Here's how the part is built. I have some questions about the finished solid (model axes, mm). A direction names the side the tool comes from. Round coordinates to 2 decimals unless told otherwise and drop trailing zeros. Order: outer loops, then holes, each group sorted by start corner. A loop starts at its lowest first (then second) coordinate and runs counter-clockwise, first axis right, second up. Notation, with made-up numbers: (18.25, 35) - (76.25, 35) arc R33 cw to (76.25, 70) - close; hole circle Ø9 at (39, 20). An arc over 180 degrees is marked (long way). One line per item, written item: value.
from build123d import *

# Parameters (mm, degrees)
SKETCH_W        = 40
SKETCH_H        = 40
PAD_DEPTH       = 2
SKETCH001_R     = 10.1
PAD001_DEPTH    = 6
SKETCH002_R     = 8
POCKET_DEPTH    = 6
SKETCH003_W     = 2.007961
SKETCH003_H     = 21.864484
SKETCH003_W_2   = 7.094803
SKETCH003_H_2   = 2.097204
SKETCH003_W_3   = 6.916317
SKETCH003_H_3   = 1.96334
POCKET001_DEPTH = 6
FILLET_R        = 2


with BuildPart() as part:
    # Sketch → Pad (new body)
    with BuildSketch(Plane.XY):
        with Locations((20, -20)):
            Rectangle(SKETCH_W, SKETCH_H)
    extrude(amount=PAD_DEPTH)

    # Sketch001 (on Face6 of Pad) → Pad001 (join)
    with BuildSketch(Plane.XY.offset(2)):
        with Locations((20, -20)):
            Circle(SKETCH001_R)
    extrude(amount=PAD001_DEPTH)

    # Sketch002 (on Face8 of Pad001) → Pocket (cut)
    with BuildSketch(Plane.XY.offset(8)):
        with Locations((20, -20)):
            Circle(SKETCH002_R)
    extrude(amount=-POCKET_DEPTH, mode=Mode.SUBTRACT)

    # Sketch003 (on Face8 of Pocket) → Pocket001 (cut)
    with BuildSketch(Plane.XY.offset(8)):
        with Locations((20.041939, -19.903789)):
            Rectangle(SKETCH003_W, SKETCH003_H)
        with Locations((28.520004, -19.970721)):
            Rectangle(SKETCH003_W_2, SKETCH003_H_2)
        with Locations((12.456301, -20.037653)):
            Rectangle(SKETCH003_W_3, SKETCH003_H_3)
    extrude(amount=-POCKET001_DEPTH, mode=Mode.SUBTRACT)

    # Fillet
    fillet_edges = [part.edges().sort_by_distance(p)[0] for p in [
        (40, -40, 1),
        (40, 0, 1),
        (0, -40, 1),
        (0, 0, 1),
    ]]
    fillet(fillet_edges, radius=FILLET_R)


solid = part.part
Q1. We'd pull the mould along Y, two halves only. Please class faces 1 (the flat face through (14, -26, 8)), 2 (the cylindrical face through (25.697, -14.384, 5.042)), 3 (the cylindrical face through (27.198, -12.915, 4.958)): released by +Y, released by -Y, zero draft, split by the parting line, or undercut.
Results list:
face 1: zero draft
face 2: undercut
face 3: released by +Y
Q2. If I drill on line 1 along Y through (x, z) = (19, 6); line 2 along Z through (x, y) = (3.5, -6.5); line 3 along X through (y, z) = (-14, 4), over which ranges is the centre line in solid material (lowest first)?
Results list:
line 1: -30.05 to -27.94, -12.06 to -9.95
line 2: 0 to 2
line 3: 11.88 to 14.71, 25.29 to 28.12
Q3. Will these pins go through, and if not, where does the flat tip stop? pin 1 (2.5 mm diameter, centred on x = 11, z = 4.5, fed in from +Y); pin 2 (2.5 mm diameter, centred on x = 28.5, z = 4.5, fed in from +Y); pin 3 (3 mm diameter, centred on y = -19, z = 4, fed in from -X).
Results list:
pin 1: y = -13.52
pin 2: y = -12.97
pin 3: x = 9.94
Q4. If we section it at B-B, the plane y = -23: Please give me the cut outline in (x, z).
Results list:
outline: (0, 0) - (40, 0) - (40, 2) - (29.64, 2) - (29.64, 8) - (27.42, 8) - (27.42, 2) - (12.58, 2) - (12.58, 8) - (10.36, 8) - (10.36, 2) - (0, 2) - close
Q5. Which directions (+Z, -Z, +X, -X, +Y, -Y) give clear straight access to the entire face, cutting with the end or side of a thin tool? Please do faces 4 (the flat face through (11, -21.019, 5)), 5 (the cylindrical face through (12.81, -27.093, 4.958)), 6 (the cylindrical face through (12.921, -12.796, 4.958)).
Results list:
face 4: +Z, +X, -X
face 5: +Z, -X, -Y
face 6: +Z, -X, +Y
Q6. If we section it at A-A, the plane z = 5.25: Please give me the cut outline in (x, y).
Results list:
outline: (9.94, -19.06) - (12.06, -19.06) arc R8 cw to (19.04, -12.06) - (19.04, -9.95) arc R10.1 ccw to start; (9.95, -21.02) arc R10.1 ccw to (19.04, -30.05) - (19.04, -27.94) arc R8 cw to (12.07, -21.02) - close; (21.05, -30.05) arc R10.1 ccw to (30.05, -21.02) - (27.93, -21.02) arc R8 cw to (21.05, -27.93) - close; (21.05, -12.07) arc R8 cw to (27.93, -18.92) - (30.04, -18.92) arc R10.1 ccw to (21.05, -9.95) - close
Q7. If we section it at C-C, the plane x = 23: Please give me the cut outline in (y, z), then the cut area to 3 significant figures.
Results list:
outline: (-40, 0) - (0, 0) - (0, 2) - (-10.36, 2) - (-10.36, 8) - (-12.58, 8) - (-12.58, 2) - (-27.42, 2) - (-27.42, 8) - (-29.64, 8) - (-29.64, 2) - (-40, 2) - close
area: 107 mm²
Q8. If we section it at D-D, the plane x = 5: Please give me the cut outline in (y, z), then the cut area to 3 significant figures.
Results list:
outline: (-40, 0) - (0, 0) - (0, 2) - (-40, 2) - close
area: 80.0 mm²
